Source: CAD feature listing. Evaluate the final solid. Frame: model axes, mm. A direction names the side the tool comes from. Give positions to 0.01 mm unless a question says otherwise; leave off trailing zeros. Write each loop counter-clockwise with the first axis right and the second up, starting at its lowest first coordinate (ties: lowest second). Pieces come first, ordered by that corner, then holes. Notation, with made-up numbers: (19.25, -21) -> (35.25, -21) arc R8 ccw to (35.25, -8) -> close; hole circle Ø1 at (64, 89). An arc over 180 degrees is marked (long way). Use one line per item in the form item = value. Start each with the question number.
(1) Cut plane A-A, the plane y = 42. Output: boundary loops of the cut face in (x, z), and give its area (3 significant figures).
(2) First-contact query: P1, Ø1.5, axis at x = 6, y = 35.5, coming from the -Z side; P2, Ø6, axis at x = -1, z = 3.5, coming from the +Y side; P3, Ø10, axis at y = 16, z = -5.5, coming from the -X side. Flat tips, straight axial feed; report the tip coordinate or a pass-through.
(3) Cut plane D-D, the plane x = -9. Output: boundary loops of the cut face in (y, z), and give its area (3 significant figures).
(4) Cut plane C-C, the plane y = 21.5. Output: boundary loops of the cut face in (x, z), and give its area (3 significant figures).
(5) Cut plane B-B, the plane z = -6. Output: boundary loops of the cut face in (x, y), and give its area (3 significant figures).
(6) Material intervals for line 1 along Y through (x, z) = (0.25, 0.5); line 2 along Z through (x, y) = (-9.25, 14); line 3 along Z through (x, y) = (10, 42), sorted ascending. Write a range as from..to.
(7) Set-up query: faces 1 (the face through (3.477, 45.93, -0.133)), 2 (the face through (0, 0, 0)). Return all of +Z, -Z, +X, -X, +Y, -Y with unobstructed straight access to the full face (end or side cutting, diameter ignored); none if empty.
(8) Draft query along X for faces 3 (the face through (0, 25, -9.5)), 4 (the face through (-0.824, 46.07, -0.133)), 5 (the face through (8.266, 25.143, -4.684)). Return one class per face: pulls with the +X half, pulls with the -X half, needs draft (parallel to the pull), parting line crosses it, or undercut.
from build123d import *

# Parameters (mm, degrees)
BOSS_EXTRUDE1_DEPTH     = 51
CUT_EXTRUDE1_DEPTH      = 54.024365468
CUT_EXTRUDE1_DEPTH_BACK = 54.024365468


with BuildPart() as part:
    # Sketch1 → Boss-Extrude1 (new body)
    with BuildSketch(Plane(origin=(0, 0, 0), x_dir=(1, 0, 0), z_dir=(0, 1, 0))):
        Polygon((-5.484827557, -9.5), (5.484827557, -9.5), (10.969655115, 0), (5.484827557, 9.5), (-5.484827557, 9.5), (-10.969655115, 0), align=None)
    extrude(amount=BOSS_EXTRUDE1_DEPTH)

    # Sketch3 → Cut-Extrude1 (cut, two sides: drawn at the far end of the back side and taken through both)
    with BuildSketch(Plane.XY.offset(-CUT_EXTRUDE1_DEPTH_BACK)):
        Polygon((-5.484827557, 51), (3.969655115, 41), (2.969655115, 51), align=None)
    extrude(amount=CUT_EXTRUDE1_DEPTH + CUT_EXTRUDE1_DEPTH_BACK, mode=Mode.SUBTRACT)


solid = part.part
Geometry says:
q1.outline = (-10.97, 0) -> (-5.48, -9.5) -> (3.02, -9.5) -> (3.02, 9.5) -> (-5.48, 9.5) -> close; (3.87, -9.5) -> (5.48, -9.5) -> (10.97, 0) -> (5.48, 9.5) -> (3.87, 9.5) -> close
q1.area = 297 mm^2
q2.P1 = -9.5
q2.P2 = 49.43
q2.P3 = -10.68
q3.outline = (0, -3.41) -> (51, -3.41) -> (51, 3.41) -> (0, 3.41) -> close
q3.area = 348 mm^2
q4.outline = (-10.97, 0) -> (-5.48, -9.5) -> (5.48, -9.5) -> (10.97, 0) -> (5.48, 9.5) -> (-5.48, 9.5) -> close
q4.area = 313 mm^2
q5.outline = (-7.51, 0) -> (7.51, 0) -> (7.51, 51) -> (2.97, 51) -> (3.97, 41) -> (-5.48, 51) -> (-7.51, 51) -> close
q5.area = 723 mm^2
q6.line_1 = 0..44.93
q6.line_2 = -2.98..2.98
q6.line_3 = -1.68..1.68
q7.face_1 = +Z, -Z
q7.face_2 = +Z, -Z, +X, -X, -Y
q8.face_3 = needs draft
q8.face_4 = undercut
q8.face_5 = pulls with the +X half
